from build123d import *

# Parameters (mm, degrees)
ESQUISSE1_W                  = 100
ESQUISSE1_H                  = 40
BOSS_EXTRU_3_DEPTH           = 70
ENL_V_MAT_EXTRU_1_DEPTH      = 92.8886174
ENL_V_MAT_EXTRU_1_DEPTH_BACK = 92.8886174
BOSS_EXTRU_5_DEPTH           = 7
BOSS_EXTRU_6_START           = 7
ESQUISSE4_W                  = 80
ESQUISSE4_H                  = 7
BOSS_EXTRU_6_DEPTH           = 7
BOSS_EXTRU_7_DEPTH           = 0.1


with BuildPart() as part:
    # Esquisse1 → Boss.-Extru.3 (new body)
    with BuildSketch(Plane.XY):
        with Locations((-2.858975564, 7.376024363)):
            Rectangle(ESQUISSE1_W, ESQUISSE1_H)
    extrude(amount=BOSS_EXTRU_3_DEPTH)

    # Esquisse2 → Enlèv. mat.-Extru.1 (cut, two sides: drawn at the far end of the back side and taken through both)
    with BuildSketch(Plane.XY.offset(70).offset(-ENL_V_MAT_EXTRU_1_DEPTH_BACK)):
        Polygon((-124.152094394, 178.669143194), (27.141024436, 27.376024363), (47.141024436, 7.376024363), (198.434143267, -143.917094467), (501.020380927, 158.669143194), (178.434143267, 481.255380855), align=None)
    extrude(amount=ENL_V_MAT_EXTRU_1_DEPTH + ENL_V_MAT_EXTRU_1_DEPTH_BACK, mode=Mode.SUBTRACT)

    # Esquisse3 → Boss.-Extru.5 (add)
    with BuildSketch(Plane(origin=(0, 0, 0), x_dir=(-1, 0, 0), z_dir=(0, 0, -1))):
        with BuildLine():
            Line((-57.141024436, -2.623975637), (-47.141024436, -12.623975637))
            Line((-47.141024436, -12.623975637), (-37.141024436, -19.623975637))
            Line((-37.141024436, -19.623975637), (42.858975564, -19.623975637))
            Line((42.858975564, -19.623975637), (52.858975564, -12.623975637))
            Line((52.858975564, -12.623975637), (62.858975564, -2.623975637))
            ThreePointArc((62.858975564, -2.623975637), (59.930043376, 4.447092175), (52.858975564, 7.376024363))
            Line((52.858975564, 7.376024363), (-47.141024436, 7.376024363))
            ThreePointArc((-47.141024436, 7.376024363), (-54.212092248, 4.447092175), (-57.141024436, -2.623975637))
        make_face()
    extrude(amount=BOSS_EXTRU_5_DEPTH)

    # Esquisse4 → Boss.-Extru.6 (add)
    with BuildSketch(Plane.XY.offset(70).offset(BOSS_EXTRU_6_START)):
        with BuildLine():
            ThreePointArc((47.141024436, 7.376024363), (54.212092248, 4.447092175), (57.141024436, -2.623975637))
            Line((57.141024436, -2.623975637), (47.141024436, -12.623975637))
            Line((47.141024436, -12.623975637), (47.141024436, 7.376024363))
        make_face()
        Polygon((47.141024436, 7.376024363), (-52.858975564, 7.376024363), (-52.858975564, -12.623975637), (-42.858975564, -12.623975637), (37.141024436, -12.623975637), (47.141024436, -12.623975637), align=None)
        Polygon((37.141024436, -19.623975637), (47.141024436, -12.623975637), (37.141024436, -12.623975637), align=None)
        with Locations((-2.858975564, -16.123975637)):
            Rectangle(ESQUISSE4_W, ESQUISSE4_H)
        Polygon((-42.858975564, -12.623975637), (-52.858975564, -12.623975637), (-42.858975564, -19.623975637), align=None)
        with BuildLine():
            Line((-52.858975564, -12.623975637), (-52.858975564, 7.376024363))
            ThreePointArc((-52.858975564, 7.376024363), (-59.930043376, 4.447092175), (-62.858975564, -2.623975637))
            Line((-62.858975564, -2.623975637), (-52.858975564, -12.623975637))
        make_face()
    extrude(amount=-BOSS_EXTRU_6_DEPTH)

    # Esquisse5 → Boss.-Extru.7 (add)
    with BuildSketch(Plane.XY.offset(77)):
        with BuildLine():
            ThreePointArc((-52.858975564, 5.997782361), (-58.856757925, 0), (-52.858975564, -5.997782361))
            Line((-52.858975564, -5.997782361), (-52.858975564, 5.997782361))
        make_face()
        with BuildLine():
            Line((-52.858975564, 5.997782361), (-52.858975564, -5.997782361))
            ThreePointArc((-52.858975564, -5.997782361), (-48.617902985, -4.241072579), (-46.861193203, 0))
            ThreePointArc((-46.861193203, 0), (-48.617902985, 4.241072579), (-52.858975564, 5.997782361))
        make_face()
    extrude(amount=BOSS_EXTRU_7_DEPTH)


solid = part.part
The listing builds one solid part. Answer for the finished solid, in the listing's coordinates (mm). A direction names the side the tool comes from. Coordinates: 2 decimals unless noted, no trailing zeros. Loops run counter-clockwise (first coordinate to the right, second up) from the corner with the lowest first, then second, coordinate; pieces in that order, holes last. Notation, with made-up numbers: (37, 79) -> (54, 79) arc R33 cw to (54, 110) -> close; hole circle Ø4 at (-23, 81). An arc over 180 degrees is marked (long way). Answer in a Markdown table with one row per item. Add a question column.
1. The part is cut by section C-C, the plane y = 4.5. Write down the section's boundary in (x, z).
2. The part is cut by section A-A, the plane z = 46. Write down the section's boundary in (x, y).
3. Flat-ended cylindrical pins translate along their axes: P1, Ø3.5, axis at x = 10, z = 74.5, coming from the +Y side; P2, Ø8, axis at y = 22, z = 28.5, coming from the -X side; P3, Ø8, axis at x = 14.5, y = -10, coming from the +Z side; P4, Ø1, axis at y = -14.5, z = 65, coming from the +X side. Find the tip coordinate at first contact, or state that the pin passes through.
4. The part is cut by section B-B, the plane x = -1. Write down the section's boundary in (y, z).
5. Determine the mould class of faces 1 (the flat face through (-4, 18, 0)), 2 (the flat face through (-2, -16, 70)), 3 (the flat face through (-4, 7.376, -3)) for opening direction Z: +Z half, -Z half, draft (parallel to the pull), parting line (faces both ways), or undercut.
6. The part is cut by section D-D, the plane x = 30. Write down the section's boundary in (y, z).
7. Consider line 1 (Y direction, x = -29, z = -1); line 2 (Z direction, x = -29, y = 3); line 3 (Y direction, x = -22.5, z = 33.5). Determine where each line is inside the solid, lowest interval first. Write a range as [from, to].
8. For faces 4 (the flat face through (-2, -16, 0)), 5 (the flat face through (-57, 0, 0)), 6 (the cylindrical face through (-60.007, 4.369, -3.451)), 7 (the flat face through (-4, 18, 70)), 8 (the flat face through (51, 0, 0)), determine the directions among +Z, -Z, +X, -X, +Y, -Y from which every point of the face is accessible in a straight line to the end or side of a thin tool.
Answer below:
| question | item | result |
|---|---|---|
| 1 | outline | (-59.88, -7) -> (54.16, -7) -> (54.16, 0) -> (47.14, 0) -> (47.14, 70) -> (54.16, 70) -> (54.16, 77) -> (-48.89, 77) -> (-48.89, 77.1) -> (-56.82, 77.1) -> (-56.82, 77) -> (-59.88, 77) -> (-59.88, 70) -> (-52.86, 70) -> (-52.86, 0) -> (-59.88, 0) -> close |
| 2 | outline | (-52.86, -12.62) -> (47.14, -12.62) -> (47.14, 7.38) -> (27.14, 27.38) -> (-52.86, 27.38) -> close |
| 3 | P1 | y = 7.38 |
| 3 | P2 | x = -52.86 |
| 3 | P3 | z = 77 |
| 3 | P4 | through |
| 4 | outline | (-19.62, -7) -> (7.38, -7) -> (7.38, 0) -> (27.38, 0) -> (27.38, 70) -> (7.38, 70) -> (7.38, 77) -> (-19.62, 77) -> (-19.62, 70) -> (-12.62, 70) -> (-12.62, 0) -> (-19.62, 0) -> close |
| 5 | face 1 | -Z half |
| 5 | face 2 | undercut |
| 5 | face 3 | draft |
| 6 | outline | (-19.62, -7) -> (7.38, -7) -> (7.38, 0) -> (24.52, 0) -> (24.52, 70) -> (7.38, 70) -> (7.38, 77) -> (-19.62, 77) -> (-19.62, 70) -> (-12.62, 70) -> (-12.62, 0) -> (-19.62, 0) -> close |
| 7 | line 1 | [-19.62, 7.38] |
| 7 | line 2 | [-7, 77] |
| 7 | line 3 | [-12.62, 27.38] |
| 8 | face 4 | +X, -X, -Y |
| 8 | face 5 | -X, +Y, -Y |
| 8 | face 6 | +Z, -Z, -X, +Y |
| 8 | face 7 | +Z, +X, -X, +Y |
| 8 | face 8 | +X, +Y, -Y |
